Could you check a few things on this model? Use its own coordinates, in mm. A direction names the side the tool comes from. Coordinates: 2 decimals unless noted, no trailing zeros. Order: outer loops, then holes, each group sorted by start corner. A loop starts at its lowest first (then second) coordinate and runs counter-clockwise, first axis right, second up. Notation, with made-up numbers: (-33, -7) - (-12, -7) arc R13 cw to (-12, 10) - close; hole circle Ø2 at (-8, 55). An arc over 180 degrees is marked (long way). Answer as a JSON object with one key per item and string values. Group by question number.
(1) Imagine slicing it at B-B, the plane y = 108. Write out the boundary of the cut face in (x, z).
(2) Will these pins go through, and if not, where does the flat tip stop? P1, Ø6, axis at x = 86, y = 42, coming from the -Z side; P2, Ø2, axis at x = 47.5, y = 77.5, coming from the -Z side; P3, Ø1.5, axis at x = 6, y = -125, coming from the +Z side; P4, Ø12, axis at x = -70, y = -149, coming from the +Z side.
(3) We'd pull the mould along X, two halves only. Please class faces 3 (the cylindrical face through (-61.13, -101.45, 7.89)), 4 (the flat face through (-100, -21, 9)), 5 (the flat face through (-1, -17, 0)): pulls with the +X half, pulls with the -X half, needs draft (parallel to the pull), parting line crosses it, or undercut.
(4) Imagine slicing it at A-A, the plane y = -149. Write out the boundary of the cut face in (x, z), and give its area (3 significant figures).
(5) Which directions (+Z, -Z, +X, -X, +Y, -Y) give clear straight access to the entire face, cutting with the end or side of a thin tool? Please do faces 1 (the conical face through (-45, 24, 1)), 2 (the flat face through (32, -21, 11)).
(6) Imagine slicing it at C-C, the plane y = 70.5. Write out the boundary of the cut face in (x, z).
(7) Please list where these lines run through material, in increasing order: probe 1 along Y at (x, z) = (-17.5, 3); probe 2 along X at (y, z) = (-12.5, 10.5); probe 3 along X at (y, z) = (55.5, 15.25).
from build123d import *

# Parameters (mm, degrees)
SKETCH1_W                      = 200
SKETCH1_H                      = 294
BOSS_EXTRUDE1_DEPTH            = 19.05
SKETCH2_W                      = 192
SKETCH2_H                      = 294
CUT_EXTRUDE1_DEPTH             = 3.05
SKETCH3_W                      = 64
SKETCH3_H                      = 294
CUT_EXTRUDE2_DEPTH             = 10
M6_CLEARANCE_HOLE1_D           = 6.6
M3X0_5_TAPPED_HOLE1_AT_2_COUNT = 2
M3X0_5_TAPPED_HOLE1_AT_2_PITCH = 19
M8_CLEARANCE_HOLE1_D           = 9
M5X0_8_TAPPED_HOLE1_D          = 4.2
MIRROR2_COPY_1_D               = 6.6
M5_CLEARANCE_HOLE1_D           = 5.5
M12X1_5_TAPPED_HOLE1_D         = 10.5


with BuildPart() as part:
    # Sketch1 → Boss-Extrude1 (new body)
    with BuildSketch(Plane.XY):
        with Locations((0, -19)):
            Rectangle(SKETCH1_W, SKETCH1_H)
    extrude(amount=BOSS_EXTRUDE1_DEPTH)

    # Sketch2 → Cut-Extrude1 (cut)
    with BuildSketch(Plane.XY.offset(19.05)):
        with Locations((4, -19)):
            Rectangle(SKETCH2_W, SKETCH2_H)
    extrude(amount=-CUT_EXTRUDE1_DEPTH, mode=Mode.SUBTRACT)

    # Sketch3 → Cut-Extrude2 (cut)
    with BuildSketch(Plane.XY.offset(16)):
        with Locations((0, -19)):
            Rectangle(SKETCH3_W, SKETCH3_H)
    extrude(amount=-CUT_EXTRUDE2_DEPTH, mode=Mode.SUBTRACT)

    # M6 Clearance Hole1 (through all)
    with Locations(Plane.XY.offset(16)):
        with Locations((54, -42), (86, -42), (86, -78), (54, -78)):
            m6_clearance_hole1 = Hole(M6_CLEARANCE_HOLE1_D / 2)

    # Mirror1: M6 Clearance Hole1 across plane
    add(m6_clearance_hole1.mirror(Plane.ZX), mode=Mode.SUBTRACT)

    # Sketch8 → M3x0.5 Tapped Hole1 (revolve, cut)
    with BuildSketch(Plane(origin=(54.5, -12.5, 16), x_dir=(0, -1, 0), z_dir=(1, 0, 0))):
        Polygon((0, 0), (0, 8.251075774), (1.25, 7.5), (1.25, 0), align=None)
    m3x0_5_tapped_hole1 = revolve(axis=Axis((54.5, -12.5, 22.35), (0, 0, -1)), mode=Mode.SUBTRACT)

    # M3x0.5 Tapped Hole1 at 2: M3x0.5 Tapped Hole1 ×2
    with Locations(*[(-i * M3X0_5_TAPPED_HOLE1_AT_2_PITCH, 0, 0) for i in range(1, M3X0_5_TAPPED_HOLE1_AT_2_COUNT)]):
        add(m3x0_5_tapped_hole1, mode=Mode.SUBTRACT)

    # Sketch10 → Ø22.5 (22.5) Diameter Hole1 (revolve, cut)
    with BuildSketch(Plane(origin=(45, 12.5, 16), x_dir=(0, -1, 0), z_dir=(1, 0, 0))):
        Polygon((0, 0), (0, 16), (12.5, 16), (11.25, 14.75), (11.25, 1.25), (12.5, 0), align=None)
    f_22_5_22_5_diameter_hole1 = revolve(axis=Axis((45, 12.5, 22.35), (0, 0, -1)), mode=Mode.SUBTRACT)

    # M8 Clearance Hole1 (through all)
    with Locations(Plane.XY.offset(16)):
        with Locations((40, 108), (80, 108)):
            m8_clearance_hole1 = Hole(M8_CLEARANCE_HOLE1_D / 2)

    # M5x0.8 Tapped Hole1 (through all)
    with Locations(Plane.XY.offset(16)):
        with Locations((40, 60), (40, -20), (40, -60)):
            m5x0_8_tapped_hole1 = Hole(M5X0_8_TAPPED_HOLE1_D / 2)

    # Mirror2: M6 Clearance Hole1, M3x0.5 Tapped Hole1, Ø22.5 (22.5) Diameter Hole1, M8 Clearance Hole1, M5x0.8 Tapped Hole1 across plane
    add(m6_clearance_hole1.mirror(Plane(origin=(0, 0, 0), x_dir=(0, 0, 1), z_dir=(1, 0, 0))), mode=Mode.SUBTRACT)
    add(m3x0_5_tapped_hole1.mirror(Plane(origin=(0, 0, 0), x_dir=(0, 0, 1), z_dir=(1, 0, 0))), mode=Mode.SUBTRACT)
    add(f_22_5_22_5_diameter_hole1.mirror(Plane(origin=(0, 0, 0), x_dir=(0, 0, 1), z_dir=(1, 0, 0))), mode=Mode.SUBTRACT)
    add(m8_clearance_hole1.mirror(Plane(origin=(0, 0, 0), x_dir=(0, 0, 1), z_dir=(1, 0, 0))), mode=Mode.SUBTRACT)
    add(m5x0_8_tapped_hole1.mirror(Plane(origin=(0, 0, 0), x_dir=(0, 0, 1), z_dir=(1, 0, 0))), mode=Mode.SUBTRACT)

    # Mirror2 copy 1 (through all)
    with Locations(Plane(origin=(0, 0, 16), x_dir=(-1, 0, 0), z_dir=(0, 0, 1))):
        with Locations((54, -42), (86, -42), (86, -78), (54, -78)):
            Hole(MIRROR2_COPY_1_D / 2)

    # Mirror2 copy 2 sketch → Mirror2 copy 2 (revolve, cut)
    with BuildSketch(Plane(origin=(-35.5, -12.5, 16), x_dir=(0, -1, 0), z_dir=(-1, 0, 0))):
        Polygon((0, 0), (0, -8.251075774), (1.25, -7.5), (1.25, 0), align=None)
    revolve(axis=Axis((-35.5, -12.5, 22.35), (0, 0, 1)), mode=Mode.SUBTRACT)

    # M5 Clearance Hole1 (through all)
    with Locations(Plane.XY.offset(6)):
        with Locations((-17.5, 22), (17.5, 22), (17.5, -2), (-17.5, -2)):
            Hole(M5_CLEARANCE_HOLE1_D / 2)

    # M12x1.5 Tapped Hole1 (through all)
    with Locations(Plane.XY.offset(16)):
        with Locations((65, -149), (-65, -105), (65, -105), (-70, -149)):
            Hole(M12X1_5_TAPPED_HOLE1_D / 2)


solid = part.part
Result set:
{
 "1": {"outline": "(-100, 0) - (-84.5, 0) - (-84.5, 16) - (-92, 16) - (-92, 19.05) - (-100, 19.05) - close; (-75.5, 0) - (-44.5, 0) - (-44.5, 16) - (-75.5, 16) - close; (-35.5, 0) - (35.5, 0) - (35.5, 16) - (32, 16) - (32, 6) - (-32, 6) - (-32, 16) - (-35.5, 16) - close; (44.5, 0) - (75.5, 0) - (75.5, 16) - (44.5, 16) - close; (84.5, 0) - (100, 0) - (100, 16) - (84.5, 16) - close"},
 "2": {"P1": "passes through", "P2": "stops at z = 0", "P3": "stops at z = 6", "P4": "stops at z = 16"},
 "3": {"face 3": "undercut", "face 4": "pulls with the -X half", "face 5": "needs draft"},
 "4": {"outline": "(-100, 0) - (-75.25, 0) - (-75.25, 16) - (-92, 16) - (-92, 19.05) - (-100, 19.05) - close; (-64.75, 0) - (59.75, 0) - (59.75, 16) - (32, 16) - (32, 6) - (-32, 6) - (-32, 16) - (-64.75, 16) - close; (70.25, 0) - (100, 0) - (100, 16) - (70.25, 16) - close", "area": "2,250 mm^2"},
 "5": {"face 1": "-Z", "face 2": "+Z, +Y, -Y"},
 "6": {"outline": "(-100, 0) - (100, 0) - (100, 16) - (32, 16) - (32, 6) - (-32, 6) - (-32, 16) - (-92, 16) - (-92, 19.05) - (-100, 19.05) - close"},
 "7": {"probe 1": "y = -166 to -4.75, 0.75 to 19.25, 24.75 to 128", "probe 2": "x = -100 to -55.75, -53.25 to -36.75, -34.25 to -32, 32 to 34.25, 36.75 to 53.25, 55.75 to 100", "probe 3": "x = -100 to -32, 32 to 100"}
}
